```python
from build123d import *

# Parameters (mm, degrees)
SKETCH1_W           = 144.5
SKETCH1_H           = 168
BOSS_EXTRUDE1_DEPTH = 2.8
CUT_EXTRUDE1_REACH  = 4.8
SKETCH2_R           = 1.55
SKETCH2_W           = 15
SKETCH2_H           = 32
CUT_EXTRUDE2_REACH  = 4.8
SKETCH5_R           = 1.55
SKETCH6_R           = 4
CUT_EXTRUDE3_DEPTH  = 1.3
CUT_EXTRUDE4_REACH  = 4.8


with BuildPart() as part:
    # Sketch1 → Boss-Extrude1 (new body)
    with BuildSketch(Plane(origin=(0, 0, 0), x_dir=(1, 0, 0), z_dir=(0, 1, 0))):
        Rectangle(SKETCH1_W, SKETCH1_H)
    extrude(amount=BOSS_EXTRUDE1_DEPTH)

    # Sketch2 → Cut-Extrude1 (cut, up to next)
    with BuildSketch(Plane(origin=(0, 2.8, 0), x_dir=(1, 0, 0), z_dir=(0, 1, 0)), mode=Mode.PRIVATE) as cut_extrude1_sk1:
        with Locations((-19.199747468, -24.95836944)):
            Circle(SKETCH2_R)
    cut_extrude1_tool1 = extrude(cut_extrude1_sk1.sketch, amount=-CUT_EXTRUDE1_REACH, mode=Mode.PRIVATE) & part.part
    add(cut_extrude1_tool1.solids().sort_by_distance((-19.199747, 2.8, 24.958369))[0], mode=Mode.SUBTRACT)
    # Sketch2 → Cut-Extrude1 (cut, up to next)
    with BuildSketch(Plane(origin=(0, 2.8, 0), x_dir=(1, 0, 0), z_dir=(0, 1, 0)), mode=Mode.PRIVATE) as cut_extrude1_sk2:
        with Locations((9.79163056, -53.949747468)):
            Circle(SKETCH2_R)
    cut_extrude1_tool2 = extrude(cut_extrude1_sk2.sketch, amount=-CUT_EXTRUDE1_REACH, mode=Mode.PRIVATE) & part.part
    add(cut_extrude1_tool2.solids().sort_by_distance((9.791631, 2.8, 53.949747))[0], mode=Mode.SUBTRACT)
    # Sketch2 → Cut-Extrude1 (cut, up to next)
    with BuildSketch(Plane(origin=(0, 2.8, 0), x_dir=(1, 0, 0), z_dir=(0, 1, 0)), mode=Mode.PRIVATE) as cut_extrude1_sk3:
        with Locations((-9.300252532, -73.04163056)):
            Circle(SKETCH2_R)
    cut_extrude1_tool3 = extrude(cut_extrude1_sk3.sketch, amount=-CUT_EXTRUDE1_REACH, mode=Mode.PRIVATE) & part.part
    add(cut_extrude1_tool3.solids().sort_by_distance((-9.300253, 2.8, 73.041631))[0], mode=Mode.SUBTRACT)
    # Sketch2 → Cut-Extrude1 (cut, up to next)
    with BuildSketch(Plane(origin=(0, 2.8, 0), x_dir=(1, 0, 0), z_dir=(0, 1, 0)), mode=Mode.PRIVATE) as cut_extrude1_sk4:
        with Locations((-38.29163056, -44.050252532)):
            Circle(SKETCH2_R)
    cut_extrude1_tool4 = extrude(cut_extrude1_sk4.sketch, amount=-CUT_EXTRUDE1_REACH, mode=Mode.PRIVATE) & part.part
    add(cut_extrude1_tool4.solids().sort_by_distance((-38.291631, 2.8, 44.050253))[0], mode=Mode.SUBTRACT)
    # Sketch2 → Cut-Extrude1 (cut, up to next)
    with BuildSketch(Plane(origin=(0, 2.8, 0), x_dir=(1, 0, 0), z_dir=(0, 1, 0)), mode=Mode.PRIVATE) as cut_extrude1_sk5:
        with Locations((64.75, 68)):
            Rectangle(SKETCH2_W, SKETCH2_H)
    cut_extrude1_tool5 = extrude(cut_extrude1_sk5.sketch, amount=-CUT_EXTRUDE1_REACH, mode=Mode.PRIVATE) & part.part
    add(cut_extrude1_tool5.solids().sort_by_distance((64.75, 2.8, -68))[0], mode=Mode.SUBTRACT)

    # Sketch5 → Cut-Extrude2 (cut, up to next)
    with BuildSketch(Plane(origin=(0, 2.8, 0), x_dir=(1, 0, 0), z_dir=(0, 1, 0)), mode=Mode.PRIVATE) as cut_extrude2_sk1:
        with Locations((12.75, 71.3)):
            Circle(SKETCH5_R)
    cut_extrude2_tool1 = extrude(cut_extrude2_sk1.sketch, amount=-CUT_EXTRUDE2_REACH, mode=Mode.PRIVATE) & part.part
    add(cut_extrude2_tool1.solids().sort_by_distance((12.75, 2.8, -71.3))[0], mode=Mode.SUBTRACT)
    # Sketch5 → Cut-Extrude2 (cut, up to next)
    with BuildSketch(Plane(origin=(0, 2.8, 0), x_dir=(1, 0, 0), z_dir=(0, 1, 0)), mode=Mode.PRIVATE) as cut_extrude2_sk2:
        with Locations((12.75, -71.3)):
            Circle(SKETCH5_R)
    cut_extrude2_tool2 = extrude(cut_extrude2_sk2.sketch, amount=-CUT_EXTRUDE2_REACH, mode=Mode.PRIVATE) & part.part
    add(cut_extrude2_tool2.solids().sort_by_distance((12.75, 2.8, 71.3))[0], mode=Mode.SUBTRACT)

    # Sketch6 → Cut-Extrude3 (cut)
    with BuildSketch(Plane(origin=(0, 2.8, 0), x_dir=(1, 0, 0), z_dir=(0, 1, 0))):
        with Locations((12.75, 71.3)):
            Circle(SKETCH6_R)
    extrude(amount=-CUT_EXTRUDE3_DEPTH, mode=Mode.SUBTRACT)

    # Sketch7 → Cut-Extrude4 (cut, up to next)
    with BuildSketch(Plane(origin=(0, 2.8, 0), x_dir=(1, 0, 0), z_dir=(0, 1, 0)), mode=Mode.PRIVATE) as cut_extrude4_sk1:
        with BuildLine():
            Line((-16.25, 84), (-16.25, 55))
            ThreePointArc((-16.25, 55), (-15.371320344, 52.878679656), (-13.25, 52))
            Line((-13.25, 52), (-5.25, 52))
            ThreePointArc((-5.25, 52), (-3.128679656, 52.878679656), (-2.25, 55))
            Line((-2.25, 55), (-2.25, 84))
            Line((-2.25, 84), (-16.25, 84))
        make_face()
    cut_extrude4_tool1 = extrude(cut_extrude4_sk1.sketch, amount=-CUT_EXTRUDE4_REACH, mode=Mode.PRIVATE) & part.part
    add(cut_extrude4_tool1.solids().sort_by_distance((-9.25, 2.8, -68.13333))[0], mode=Mode.SUBTRACT)


solid = part.part
```
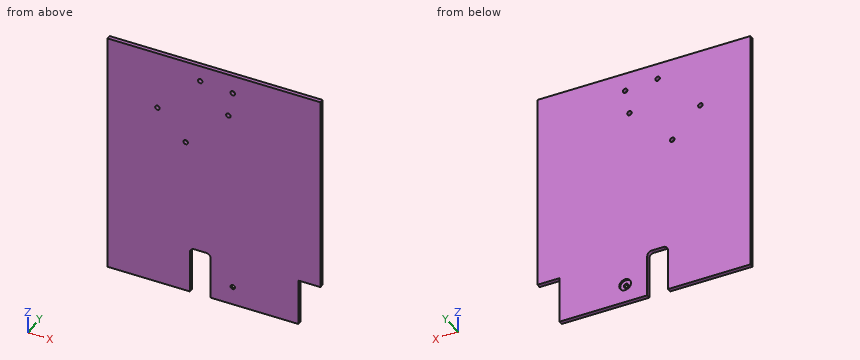
The model under review builds one solid part; all positions refer to its coordinate system, in mm. Round coordinates to 2 decimals unless told otherwise and drop trailing zeros. Loops run counter-clockwise (first coordinate to the right, second up) from the corner with the lowest first, then second, coordinate; pieces in that order, holes last. Notation, with made-up numbers: (-32.75, -34) -> (-9.75, -34) arc R32 ccw to (-9.75, -5) -> close; hole circle Ø10 at (-12.75, 86.5). An arc over 180 degrees is marked (long way). Answer in a Markdown table with one row per item.
1) Wall thickness on line 1 along Z through (x, y) = (12.75, 0.5); line 2 along X through (y, z) = (1.8, -75); line 3 along X through (y, z) = (1.3, -61): over which ranges is each line inside the solid? List them lowest first.
Taken from the geometry:
| item | result |
|---|---|
| line 1 | z = -84 to -72.85, -69.75 to 69.75, 72.85 to 84 |
| line 2 | x = -72.25 to -16.25, -2.25 to 11.23, 14.27 to 57.25 |
| line 3 | x = -72.25 to -16.25, -2.25 to 57.25 |
2) For pin 1 Ø5 at (x, z) = (12.75, -71.3) entering from +Y, flat-tipped, find the tip position at first contact; note if it passes through.
Taken from the geometry:
| item | result |
|---|---|
| pin 1 | stops at y = 1.5 |
3) Consider section B-B, the plane x = 61.5. Write out the cut boundary in (y, z).
Taken from the geometry:
| item | result |
|---|---|
| outline | (0, -52) -> (2.8, -52) -> (2.8, 84) -> (0, 84) -> close |
4) Consider section A-A, the plane y = 0.7. Write out the cut boundary in (x, z), plus the area to 3 significant figures.
Taken from the geometry:
| item | result |
|---|---|
| outline | (-72.25, -84) -> (-16.25, -84) -> (-16.25, -55) arc R3 cw to (-13.25, -52) -> (-5.25, -52) arc R3 cw to (-2.25, -55) -> (-2.25, -84) -> (57.25, -84) -> (57.25, -52) -> (72.25, -52) -> (72.25, 84) -> (-72.25, 84) -> close; hole circle Ø3.1 at (-38.29, 44.05); hole circle Ø3.1 at (-19.2, 24.96); hole circle Ø3.1 at (-9.3, 73.04); hole circle Ø3.1 at (9.79, 53.95); hole circle Ø3.1 at (12.75, -71.3); hole circle Ø3.1 at (12.75, 71.3) |
| area | 23,300 mm² |
